Design review of the part built by this model. Coordinates are the model's own, in mm. A direction names the side the tool comes from. Coordinates: 2 decimals unless noted, no trailing zeros. Write each loop counter-clockwise with the first axis right and the second up, starting at its lowest first coordinate (ties: lowest second). Pieces come first, ordered by that corner, then holes.
Q1. The part is to be moulded in two halves that separate along X. For faces 1 (the face through (-65, -14, -20)), 2 (the face through (-12, -21, -12)), 3 (the face through (-61.398, -16.784, -22.233)), say which applies: +X half, -X half, draft (parallel to the pull), parting line (faces both ways), or undercut.
Q2. To check wall thickness, follow probe 1 along X at (y, z) = (-13, -4.25); probe 2 along X at (y, z) = (-8.5, -22.25); probe 3 along X at (y, z) = (-13.5, -23.25). State the ranges of each line that lie inside material, in increasing order.
Q3. Add section D-D, the plane x = -46. Give the boundary of the cut face in (y, z).
Q4. Add section B-B, the plane y = -32.5. Give the boundary of the cut face in (x, z).
Q5. Add section A-A, the plane z = -22.5. Give the boundary of the cut face in (x, y), plus the area to 3 significant figures.
Q6. Machinability: for faces 4 (the face through (-62.04, -15.13, -22.39)), 5 (the face through (-97, 8, -17)), which of the approach directions +Z, -Z, +X, -X, +Y, -Y give a long, thin tool a straight path to every point of the face, cutting with its end or side? Answer none if there is none.
Q7. Add section C-C, the plane z = -18.5. Give the boundary of the cut face in (x, y), plus the area to 3 significant figures.
Q8. Clearance check with flat-ended pins moving along their axes: pin 1 Ø0.8 at (x, z) = (-11.5, -12.5) entering from +Y; pin 2 Ø4 at (y, z) = (0, -16.5) entering from -X; pin 3 Ø0.5 at (y, z) = (-42.5, -10.5) entering from -X. State where each tip first meets the part, or that it passes through.
from build123d import *

# Parameters (mm, degrees)
EXTRUDE018_DEPTH = 60
EXTRUDE016_DEPTH = 26.5


with BuildPart() as body013:
    # Sketch022 → Extrude018 (new body)
    with BuildSketch(Plane.XZ.offset(46)):
        Polygon((-21, 7.5), (-102, 7.5), (-102, -12), (-94, -20), (-26, -20), (-21, -15), align=None)
    extrude(amount=-EXTRUDE018_DEPTH)


with BuildPart() as cut008:
    # Sketch020 → Extrude016 (new body)
    with BuildSketch(Plane.XY.offset(-25.5)):
        Polygon((-11, 0), (-11, -43), (-23.310892, -43), (-100.566983, 10.17627), (-100, 11), (-23, -42), (-12, -42), (-12, 0), align=None)
    extrude(amount=EXTRUDE016_DEPTH)

    # Cut008: cut Body013
    add(body013.part, mode=Mode.SUBTRACT)


solid = cut008.part
Here are the results:
1. face 1: draft
1. face 2: undercut
1. face 3: -X half
2. probe 1: x = -12 to -11
2. probe 2: x = -73.43 to -71.67, -12 to -11
2. probe 3: x = -66.17 to -64.41, -12 to -11
3. outline: (-27.38, -25.5) - (-26.17, -25.5) - (-26.17, -20) - (-27.38, -20) - close
4. outline: (-38.57, -25.5) - (-36.8, -25.5) - (-36.8, -20) - (-38.57, -20) - close; (-12, -25.5) - (-11, -25.5) - (-11, 1) - (-12, 1) - close
5. outline: (-100.57, 10.18) - (-23.31, -43) - (-11, -43) - (-11, 0) - (-12, 0) - (-12, -42) - (-23, -42) - (-100, 11) - close
5. area: 148 mm2
6. face 4: +Z, -Z, +Y
6. face 5: +Z, +X, +Y, -Y
7. outline: (-100.57, 10.18) - (-95.5, 6.69) - (-95.5, 7.9) - (-100, 11) - close; (-24.5, -42.18) - (-23.31, -43) - (-11, -43) - (-11, 0) - (-12, 0) - (-12, -42) - (-23, -42) - (-24.5, -40.97) - close
7. area: 61.6 mm2
8. pin 1: stops at y = 0
8. pin 2: stops at x = -12
8. pin 3: stops at x = -21
